Input: part model. Units: mm. Frame: model coordinates. Face numbers are marked on the shaded views. Round coordinates to 2 decimals unless told otherwise and drop trailing zeros. Loops run counter-clockwise (first coordinate to the right, second up) from the corner with the lowest first, then second, coordinate; pieces in that order, holes last.
(1) Draft query along Y for the marked faces 1, 2 and 3. Return one class per face: released by +Y, released by -Y, zero draft, split by the parting line, or undercut.
(2) Cut plane C-C, the plane x = 6. Output: boundary loops of the cut face in (y, z).
(3) Cut plane B-B, the plane x = 10.75. Output: boundary loops of the cut face in (y, z).
(4) Cut plane A-A, the plane y = -17. Output: boundary loops of the cut face in (x, z).
(5) First-contact query: pin 1 Ø0.6 at (x, z) = (6, 0.5) entering from -Y; pin 2 Ø0.6 at (y, z) = (-3, 1) entering from -X; pin 3 Ø7.5 at (x, y) = (2, -15.5) entering from -Z. Flat tips, straight axial feed; report the tip coordinate or a pass-through.
(6) Cut plane D-D, the plane y = -1.5. Output: boundary loops of the cut face in (x, z).
(7) Line query: line 1 (X direction, y = -17, z = 4.55); line 2 (Z direction, x = -5.25, y = -15); line 3 (X direction, y = -17.5, z = 6). Output: solid intervals per line, ascending.
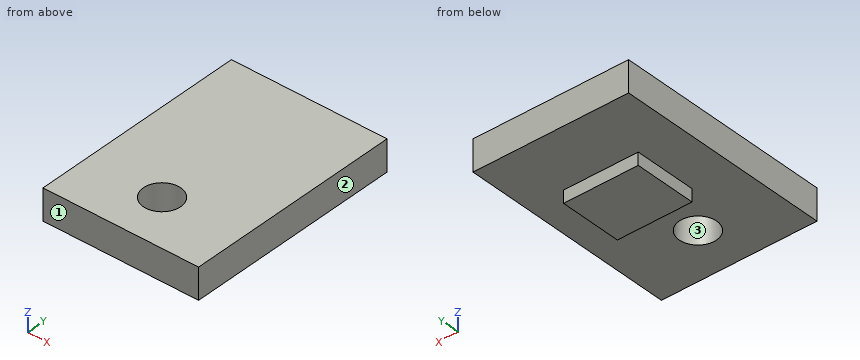
from build123d import *

# Parameters (mm, degrees)
SKIZZE1_W                            = 12
SKIZZE1_H                            = 10
HALTERUNGSSOCKEL_DEPTH               = 2
SKIZZE2_W                            = 25
SKIZZE2_H                            = 35
AUFSATZ_LINEAR_AUSTRAGEN2_DEPTH      = 5
SCHNITT_LINEAR_AUSTRAGEN1_DEPTH      = 32.533266888
SCHNITT_LINEAR_AUSTRAGEN1_DEPTH_BACK = 32.533266888
SKIZZE3_R                            = 3


with BuildPart() as part:
    # Skizze1 → Halterungssockel (new body)
    with BuildSketch(Plane.XY):
        with Locations((6, -5)):
            Rectangle(SKIZZE1_W, SKIZZE1_H)
    extrude(amount=HALTERUNGSSOCKEL_DEPTH)

    # Skizze2 → Aufsatz-Linear austragen2 (add)
    with BuildSketch(Plane.XY.offset(2)):
        with Locations((5.39823792, -7.5)):
            Rectangle(SKIZZE2_W, SKIZZE2_H)
    extrude(amount=AUFSATZ_LINEAR_AUSTRAGEN2_DEPTH)

    # Skizze3 → Schnitt-Linear austragen1 (cut, two sides: drawn at the far end of the back side and taken through both)
    with BuildSketch(Plane(origin=(0, 0, 0), x_dir=(-1, 0, 0), z_dir=(0, 0, -1)).offset(-SCHNITT_LINEAR_AUSTRAGEN1_DEPTH_BACK)):
        with Locations((-5.108390275, -17)):
            Circle(SKIZZE3_R)
    extrude(amount=SCHNITT_LINEAR_AUSTRAGEN1_DEPTH + SCHNITT_LINEAR_AUSTRAGEN1_DEPTH_BACK, mode=Mode.SUBTRACT)


solid = part.part
Reported:
1. face 1: released by -Y
1. face 2: zero draft
1. face 3: undercut
2. outline: (-25, 2) - (-19.86, 2) - (-19.86, 7) - (-25, 7) - close; (-14.14, 2) - (-10, 2) - (-10, 0) - (0, 0) - (0, 2) - (10, 2) - (10, 7) - (-14.14, 7) - close
3. outline: (-25, 2) - (-10, 2) - (-10, 0) - (0, 0) - (0, 2) - (10, 2) - (10, 7) - (-25, 7) - close
4. outline: (-7.1, 2) - (2.11, 2) - (2.11, 7) - (-7.1, 7) - close; (8.11, 2) - (17.9, 2) - (17.9, 7) - (8.11, 7) - close
5. pin 1: stops at y = -10
5. pin 2: stops at x = 0
5. pin 3: stops at z = 2
6. outline: (-7.1, 2) - (0, 2) - (0, 0) - (12, 0) - (12, 2) - (17.9, 2) - (17.9, 7) - (-7.1, 7) - close
7. line 1: x = -7.1 to 2.11, 8.11 to 17.9
7. line 2: z = 2 to 7
7. line 3: x = -7.1 to 2.15, 8.07 to 17.9
